Here's how the part is built. I have some questions about the finished solid (model axes, mm). Face numbers are marked on the shaded views. A direction names the side the tool comes from. Coordinates: 2 decimals unless noted, no trailing zeros. Write each loop counter-clockwise with the first axis right and the second up, starting at its lowest first coordinate (ties: lowest second). Pieces come first, ordered by that corner, then holes. Notation, with made-up numbers: (39.25, -13) -> (55.25, -13) arc R11 cw to (55.25, -5) -> close; hole circle Ø4 at (-19, 38.25). An arc over 180 degrees is marked (long way). Use a Markdown table: item, result. Add a question column.
Item 1: Imagine slicing it at D-D, the plane x = 0. Write out the boundary of the cut face in (y, z) (1 decimal).
Item 2: Imagine slicing it at C-C, the plane z = 2.25. Count the separate pieces of the cut face and the enclosed holes in it, and give its area (3 significant figures).
Item 3: If I drill on line 1 along X through (y, z) = (-16, 8.5); line 2 along Y through (x, z) = (-7, 0.75); line 3 along Y through (x, z) = (13.5, 1.75), over which ranges is the centre line in solid material (lowest first)? Write a range as from..to.
Item 4: Imagine slicing it at A-A, the plane y = 0. Write out the boundary of the cut face in (x, z) (1 decimal).
Item 5: If we mould it in two halves opening along Y, with no side actions, what happens to the marked faces 3, 4 and 5? For each: pulls with the +Y half, pulls with the -Y half, needs draft (parallel to the pull), parting line crosses it, or undercut.
Item 6: On a 3-axis mill with a long thin cutter (end or side, diameter ignored), from which of +Z, -Z, +X, -X, +Y, -Y can I reach the whole of each face in a straight line? I mean the marked faces 1 and 2. Say none if no direction works.
Item 7: Imagine slicing it at B-B, the plane x = -6. Write out the boundary of the cut face in (y, z).
Item 8: Will these pins go through, and if not, where does the flat tip stop? pin 1 Ø5 at (x, z) = (-1.5, 6) entering from -Y (3 decimals); pin 2 Ø3 at (x, z) = (16, 7) entering from +Y; pin 3 Ø3 at (y, z) = (-15.5, 9.5) entering from -X; pin 4 Ø2.5 at (x, y) = (14.67, 6.08) entering from -Z.
```python
from build123d import *

# Parameters (mm, degrees)
F3_DEPTH = 12.7
F4_R     = 0.508
F2_R     = 1.5875
F5_DEPTH = 12.7


# Not quite as in the source:
# - a variable given as a bare number and used for a length is read in inches; the dataset says mm whatever the document's units were


with BuildPart() as f3:
    # F1 (on Top) → F3 (new body)
    with BuildSketch(Plane.XY):
        with BuildLine():
            Line((-7.3025, 4.3464899063), (-7.3025, 20.9910485386))
            ThreePointArc((-7.3025, 20.9910485386), (0, -22.225), (7.3025, 20.9910485386))
            Line((7.3025, 20.9910485386), (7.3025, 4.3464899063))
            Line((7.3025, 4.3464899063), (6.7952360256, 3.8508022029))
            ThreePointArc((6.7952360256, 3.8508022029), (0, -7.8105), (-6.7952360256, 3.8508022029))
            Line((-6.7952360256, 3.8508022029), (-7.3025, 4.3464899063))
        make_face()
    extrude(amount=F3_DEPTH)

    # F4
    f4_edges = [f3.edges().sort_by_distance(p)[0] for p in [
        (-6.795236, 3.850802, 6.35),
        (6.795236, 3.850802, 6.35),
        (-7.3025, 20.991049, 6.35),
        (7.3025, 20.991049, 6.35),
    ]]
    fillet(f4_edges, radius=F4_R)

    # F2 (on Top) → F5 (cut, through all)
    with BuildSketch(Plane.XY):
        with Locations((-14.6665875786, 6.0750994888)):
            Circle(F2_R)
        with Locations((-14.6665875786, -6.0750994888)):
            Circle(F2_R)
        with Locations((-6.0750994888, -14.6665875786)):
            Circle(F2_R)
        with Locations((6.0750994888, -14.6665875786)):
            Circle(F2_R)
        with Locations((14.6665875786, -6.0750994888)):
            Circle(F2_R)
        with Locations((14.6665875786, 6.0750994888)):
            Circle(F2_R)
    extrude(amount=F5_DEPTH, mode=Mode.SUBTRACT)


solid = f3.part
```
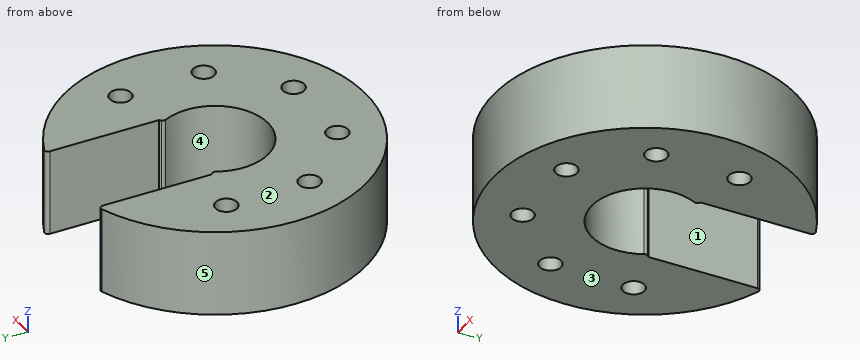
Ans:
| question | item | result |
|---|---|---|
| 1 | outline | (-22.2, 0) -> (-7.8, 0) -> (-7.8, 12.7) -> (-22.2, 12.7) -> close |
| 2 | separate pieces | 1 |
| 2 | enclosed holes | 6 |
| 2 | area | 1,090 mm^2 |
| 3 | line 1 | x = -15.43..-6.94, -5.21..5.21, 6.94..15.43 |
| 3 | line 2 | y = -21.09..-15.96, -13.38..-3.46, 3.46..4.04 |
| 3 | line 3 | y = -17.66..-7.15, -5..5, 7.15..17.66 |
| 4 | outline | (-22.2, 0) -> (-7.8, 0) -> (-7.8, 12.7) -> (-22.2, 12.7) -> close; (7.8, 0) -> (22.2, 0) -> (22.2, 12.7) -> (7.8, 12.7) -> close |
| 5 | face 3 | needs draft |
| 5 | face 4 | undercut |
| 5 | face 5 | parting line crosses it |
| 6 | face 1 | +Z, -Z, +Y |
| 6 | face 2 | +Z, +X, -X, +Y, -Y |
| 7 | outline | (-21.4, 0) -> (-16.25, 0) -> (-16.25, 12.7) -> (-21.4, 12.7) -> close; (-13.08, 0) -> (-5, 0) -> (-5, 12.7) -> (-13.08, 12.7) -> close |
| 8 | pin 1 | stops at y = -22.225 |
| 8 | pin 2 | stops at y = 16.84 |
| 8 | pin 3 | stops at x = -17.26 |
| 8 | pin 4 | passes through |
